The listing builds one solid part. Answer for the finished solid, in the listing's coordinates (mm). Give positions to 0.01 mm unless a question says otherwise; leave off trailing zeros. Loops run counter-clockwise (first coordinate to the right, second up) from the corner with the lowest first, then second, coordinate; pieces in that order, holes last. Notation, with made-up numbers: (70, 36.25) - (112, 36.25) arc R27 ccw to (112, 63.25) - close; hole circle Ø6 at (-2.5, 69). An arc over 180 degrees is marked (long way). One line per item, written item: value. Start each with the question number.
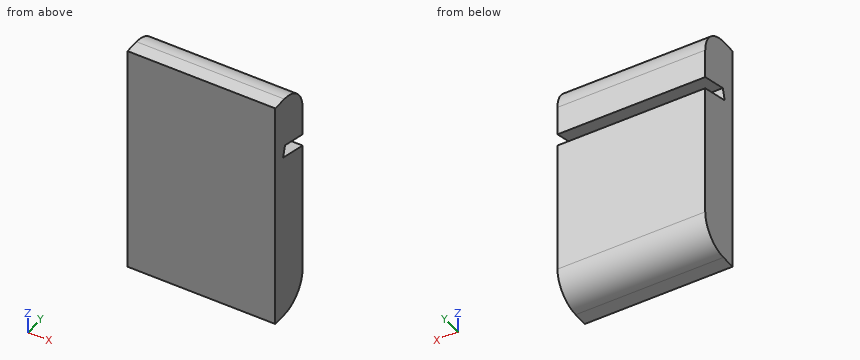
from build123d import *

# Parameters (mm, degrees)
BOSS_EXTRU_1_DEPTH = 50
CONG_1_R           = 10


with BuildPart() as part:
    # Esquisse1 → Boss.-Extru.1 (new body)
    with BuildSketch(Plane(origin=(0, 0, 0), x_dir=(0, 0, -1), z_dir=(1, 0, 0))):
        Polygon((-40, 0), (40, 0), (40, 15), (-15.858895278, 15), (-18.724487146, 4.305465557), (-22.588190451, 5.340741737), (-20, 15), (-40, 15), align=None)
    extrude(amount=BOSS_EXTRU_1_DEPTH)

    # Congé1
    cong_1_edges = [part.edges().sort_by_distance(p)[0] for p in [
        (25, 15, -40),
        (25, 15, 40),
    ]]
    fillet(cong_1_edges, radius=CONG_1_R)


solid = part.part
1. A cutting plane is placed at A-A (y = 14). Determine the outline of the cut face in (x, z), plus the area to 3 significant figures.
2. A cutting plane is placed at B-B (x = 29.5). Determine the outline of the cut face in (y, z).
3. A cutting plane is placed at D-D (z = 35). Determine the outline of the cut face in (x, y), plus the area to 3 significant figures.
4. A cutting plane is placed at C-C (y = 7). Determine the outline of the cut face in (x, z).
5. Find the intervals of material crossed by L1, parallel to Z at x = 22, y = 10.75; L2, parallel to Z at x = 39.5, y = 7.75; L3, parallel to Y at x = 43.5, z = -34, in increasing order. Write a range as [from, to].
6. Flat-ended cylindrical pins translate along their axes: pin 1 (6 mm diameter, centred on y = 12.5, z = 5, fed in from -X); pin 2 (8 mm diameter, centred on x = 16.5, y = 13, fed in from -Z); pin 3 (6 mm diameter, centred on x = 33.5, y = 9, fed in from -Z). Find the tip coordinate at first contact, or state that the pin passes through.
Results below:
1. outline: (0, -34.36) - (50, -34.36) - (50, 16.13) - (0, 16.13) - close; (0, 20.27) - (50, 20.27) - (50, 34.36) - (0, 34.36) - close
1. area: 3,230 mm^2
2. outline: (0, -40) - (5, -40) arc R10 ccw to (15, -30) - (15, 15.86) - (4.31, 18.72) - (5.34, 22.59) - (15, 20) - (15, 30) arc R10 ccw to (5, 40) - (0, 40) - close
3. outline: (0, 0) - (50, 0) - (50, 13.66) - (0, 13.66) - close
3. area: 683 mm^2
4. outline: (0, -39.8) - (50, -39.8) - (50, 18) - (0, 18) - close; (0, 22.14) - (50, 22.14) - (50, 39.8) - (0, 39.8) - close
5. L1: z = [-38.18, 17], [21.14, 38.18]
5. L2: z = [-39.61, 17.8], [21.94, 39.61]
5. L3: y = [0, 14.17]
6. pin 1: stops at x = 0
6. pin 2: stops at z = -39.17
6. pin 3: stops at z = -39.95
